```python
from build123d import *

# Parameters (mm, degrees)
SKETCH1_W           = 647.7
SKETCH1_H           = 1663.7
BOSS_EXTRUDE1_DEPTH = 26.162
SKETCH2_W           = 546.1
SKETCH2_H           = 1612.9
CUT_EXTRUDE1_DEPTH  = 26.162
CUT_EXTRUDE2_DEPTH  = 26.162
CUT_EXTRUDE3_DEPTH  = 24.13
FILLET1_R           = 12.7
SHELL4_START        = 1.778
SHELL4_DEPTH        = 22.606


# Read off the part's stored shape, not the designer's step: Shell4
with BuildPart() as part:
    # Sketch1 → Boss-Extrude1 (new body)
    with BuildSketch(Plane.XY):
        Rectangle(SKETCH1_W, SKETCH1_H)
    extrude(amount=BOSS_EXTRUDE1_DEPTH)

    # Sketch2 → Cut-Extrude1 (cut)
    with BuildSketch(Plane.XY.offset(26.162)):
        with Locations((0, -25.4)):
            Rectangle(SKETCH2_W, SKETCH2_H)
    extrude(amount=-CUT_EXTRUDE1_DEPTH, mode=Mode.SUBTRACT)

    # Sketch3 → Cut-Extrude2 (cut)
    with BuildSketch(Plane.XY.offset(26.162)):
        with BuildLine():
            Line((-317.951280605, 813.251280605), (-273.05, 768.35))
            Line((-273.05, 768.35), (-273.05, 781.05))
            Line((-273.05, 781.05), (-260.35, 781.05))
            Line((-260.35, 781.05), (-305.950453026, 825.241047594))
            ThreePointArc((-305.950453026, 825.241047594), (-317.94851482, 825.249344949), (-317.951280605, 813.251280605))
        make_face()
        with BuildLine():
            Line((305.950453026, 825.241047594), (260.35, 781.05))
            Line((260.35, 781.05), (273.05, 781.05))
            Line((273.05, 781.05), (273.05, 768.35))
            Line((273.05, 768.35), (317.951280605, 813.251280605))
            ThreePointArc((317.951280605, 813.251280605), (317.94851482, 825.249344949), (305.950453026, 825.241047594))
        make_face()
    extrude(amount=-CUT_EXTRUDE2_DEPTH, mode=Mode.SUBTRACT)

    # Sketch4 → Cut-Extrude3 (cut)
    with BuildSketch(Plane(origin=(0, 0, 0), x_dir=(-1, 0, 0), z_dir=(0, 0, -1))):
        Polygon((-307.8988, 768.35), (-307.8988, 803.1988), (-273.05, 768.35), (-273.05, -831.85), (-307.8988, -831.85), align=None)
        Polygon((-260.35, 781.05), (-295.735951532, 815.342252918), (295.735951532, 815.342252918), (260.35, 781.05), align=None)
        Polygon((307.8988, 803.1988), (273.05, 768.35), (273.05, -831.85), (307.8988, -831.85), (307.8988, 768.35), align=None)
    extrude(amount=-CUT_EXTRUDE3_DEPTH, mode=Mode.SUBTRACT)

    # Fillet1
    fillet1_edges = [part.edges().sort_by_distance(p)[0] for p in [
        (-323.85, 831.85, 13.081),
        (323.85, 831.85, 13.081),
    ]]
    fillet(fillet1_edges, radius=FILLET1_R)

    # Shell4 outline → Shell4 (cut)
    with BuildSketch(Plane.XY.offset(SHELL4_START)):
        with BuildLine():
            Line((307.8988, 803.1988), (307.8988, -830.072))
            Line((307.8988, -830.072), (322.072, -830.072))
            Line((322.072, -830.072), (322.072, 817.550302353))
            ThreePointArc((322.072, 817.550302353), (321.07369087, 814.548798877), (319.208516462, 811.994044748))
            Line((319.208516462, 811.994044748), (317.951280605, 813.251280605))
            Line((317.951280605, 813.251280605), (307.8988, 803.1988))
        make_face()
        with BuildLine():
            Line((-322.072, -830.072), (-307.8988, -830.072))
            Line((-307.8988, -830.072), (-307.8988, 803.1988))
            Line((-307.8988, 803.1988), (-317.951280605, 813.251280605))
            Line((-317.951280605, 813.251280605), (-319.208516462, 811.994044748))
            ThreePointArc((-319.208516462, 811.994044748), (-321.07369087, 814.548798877), (-322.072, 817.550302353))
            Line((-322.072, 817.550302353), (-322.072, -830.072))
        make_face()
        with BuildLine():
            ThreePointArc((301.905011396, 821.320641288), (309.142763578, 829.116339567), (319.402097182, 826.304926702))
            ThreePointArc((319.402097182, 826.304926702), (315.685635268, 829.085698099), (311.15, 830.072))
            Line((311.15, 830.072), (-311.15, 830.072))
            ThreePointArc((-311.15, 830.072), (-315.685635267, 829.085698099), (-319.402097181, 826.304926702))
            ThreePointArc((-319.402097181, 826.304926702), (-309.142763577, 829.116339567), (-301.905011396, 821.320641288))
            Line((-301.905011396, 821.320641288), (-295.735951532, 815.342252918))
            Line((-295.735951532, 815.342252918), (295.735951532, 815.342252918))
            Line((295.735951532, 815.342252918), (301.905011396, 821.320641288))
        make_face()
    extrude(amount=SHELL4_DEPTH, mode=Mode.SUBTRACT)


solid = part.part
```
The model under review builds one solid part; all positions refer to its coordinate system, in mm. A direction names the side the tool comes from. Round coordinates to 2 decimals unless told otherwise and drop trailing zeros. Loops run counter-clockwise (first coordinate to the right, second up) from the corner with the lowest first, then second, coordinate; pieces in that order, holes last. Notation, with made-up numbers: (-31.5, 9) - (-23.5, 9) arc R22 cw to (-23.5, 24) - close; hole circle Ø8 at (58.5, 78). An arc over 180 degrees is marked (long way). Write each question's results on one line, items separated by ' | '. Start each with the question number.
Q1. Take a section at C-C on x = 134. Give the boundary of the cut face in (y, z).
Q2. Wall thickness on line 1 along X through (y, z) = (-707.5, 22.75); line 2 along Y through (x, z) = (25.5, 16.5); line 3 along Z through (x, y) = (297.5, -308): over which ranges is each line inside the solid? List them lowest first. Write a range as [from, to].
Q3. Insertion check: P1, Ø11.5, axis at x = -315, y = 381, coming from the -Z side; P2, Ø2, axis at x = 53.5, z = 25, coming from the -Y side; P3, Ø2, axis at x = 136, z = 1, coming from the -Y side; P4, Ø6, axis at x = 104.5, z = 20, coming from the -Y side. Each pin has a flat end and moves straight along its axis. Give the tip position at first contact, or say it passes through.
Q4. Tool access review of faces 1 (the flat face through (-295.8, 791.1, 25.2)), 2 (the flat face through (-289, 66, 26.162)), 3 (the flat face through (-290, -3, 24.13)): name each direction out of +Z, -Z, +X, -X, +Y, -Y from which nothing blocks a thin tool from reaching the whole face with its end or side.
Q5. Draft analysis for pull direction X (two halves, no side actions). For faces 4 (the flat face through (-313, 4, 0)), 5 (the flat face through (290, -3, 24.13)), state which applies: pulls with the +X half, pulls with the -X half, needs draft (parallel to the pull), parting line crosses it, or undercut.
Q6. Take a section at B-B on z = 10. Give the boundary of the cut face in (x, y).
Q7. Take a section at A-A on y = 75.5. Give the boundary of the cut face in (x, z), plus the area to 3 significant figures.
Data:
1) outline: (781.05, 24.13) - (815.34, 24.13) - (815.34, 24.38) - (830.07, 24.38) - (830.07, 1.78) - (815.34, 1.78) - (815.34, 0) - (831.85, 0) - (831.85, 26.16) - (781.05, 26.16) - close
2) line 1: x = [-323.85, -322.07], [322.07, 323.85] | line 2: y = [830.07, 831.85] | line 3: z = [24.13, 26.16]
3) P1: stops at z = 0 | P2: stops at y = 781.05 | P3: stops at y = 815.34 | P4: stops at y = 830.07
4) face 1: +Z, -Z | face 2: +Z, +X, -X, +Y, -Y | face 3: -Z, -Y
5) face 4: needs draft | face 5: undercut
6) outline: (-323.85, -831.85) - (-307.9, -831.85) - (-307.9, -830.07) - (-322.07, -830.07) - (-322.07, 817.55) arc R10.26 ccw to (-319.21, 811.99) - (-317.95, 813.25) arc R8.48 cw to (-305.95, 825.24) - (-301.91, 821.32) arc R10.26 ccw to (-319.4, 826.3) arc R10.92 cw to (-311.15, 830.07) - (311.15, 830.07) arc R10.92 cw to (319.4, 826.3) arc R10.26 ccw to (301.91, 821.32) - (305.95, 825.24) arc R8.48 cw to (317.95, 813.25) - (319.21, 811.99) arc R10.26 ccw to (322.07, 817.55) - (322.07, -830.07) - (307.9, -830.07) - (307.9, -831.85) - (323.85, -831.85) - (323.85, 819.15) arc R12.7 ccw to (311.15, 831.85) - (-311.15, 831.85) arc R12.7 ccw to (-323.85, 819.15) - close
7) outline: (-323.85, 0) - (-307.9, 0) - (-307.9, 1.78) - (-322.07, 1.78) - (-322.07, 24.38) - (-307.9, 24.38) - (-307.9, 24.13) - (-273.05, 24.13) - (-273.05, 26.16) - (-323.85, 26.16) - close; (273.05, 24.13) - (307.9, 24.13) - (307.9, 24.38) - (322.07, 24.38) - (322.07, 1.78) - (307.9, 1.78) - (307.9, 0) - (323.85, 0) - (323.85, 26.16) - (273.05, 26.16) - close | area: 335 mm²
